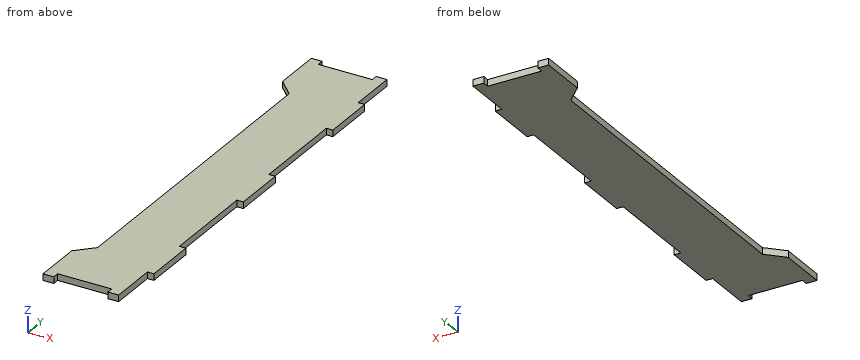
Autodesk Inventor part; units mm, degrees
ref_plane "YZ Plane" through (0, 0, 0) normal (1, 0, 0) x (0, 1, 0)
ref_plane "XZ Plane" through (0, 0, 0) normal (0, 1, 0) x (-1, 0, 0)
ref_plane "XY Plane" through (0, 0, 0) normal (0, 0, 1) x (1, 0, 0)
sketch "Sketch1" plane through (0, 0, 0) normal (0, 0, 1) x (1, 0, 0)
  line L0 (-6, 375) -> (0, 375) construction
  line L1 (0, 375) -> (0, 420) construction
  line L2 (0, 420) -> (-6, 420) construction
  line L3 (-6, 375) -> (-6, 420) construction
  line L4 (-6, 235) -> (0, 235) construction
  line L5 (0, 235) -> (0, 325) construction
  line L6 (0, 325) -> (-6, 325) construction
  line L7 (-6, 235) -> (-6, 325) construction
  line L8 (0, 185) -> (-6, 185) construction
  line L9 (-6, 95) -> (-6, 185) construction
  line L10 (-6, 95) -> (0, 95) construction
  line L11 (0, 95) -> (0, 185) construction
  line L12 (0, 45) -> (-6, 45) construction
  line L13 (-6, 0) -> (-6, 45) construction
  line L14 (0, 0) -> (-6, 0) construction
  line L15 (0, 0) -> (0, 45) construction
  line L16 (-6, 375) -> (0, 375)
  line L17 (0, 375) -> (0, 325)
  line L18 (0, 325) -> (-6, 325)
  line L19 (-6, 235) -> (0, 235)
  line L20 (0, 235) -> (0, 185)
  line L21 (0, 185) -> (-6, 185)
  line L22 (-6, 95) -> (0, 95)
  line L23 (0, 95) -> (0, 45)
  line L24 (0, 45) -> (-6, 45)
  line L25 (-6, 0) -> (-6, 45)
  line L26 (-6, 95) -> (-6, 185)
  line L27 (-6, 235) -> (-6, 325)
  line L28 (-6, 375) -> (-6, 420)
  line L29 (-76, 375) -> (-61, 375)
  line L30 (-61, 375) -> (-61, 45)
  line L31 (-61, 45) -> (-76, 45)
  line L32 (-76, 420) -> (-76, 375)
  line L33 (-76, 45) -> (-76, 0)
  line L34 (-66, 420) -> (-66, 414)
  line L35 (-66, 414) -> (-16, 414)
  line L36 (-16, 414) -> (-16, 420)
  line L37 (0, 210) -> (-61, 210) construction
  line L38 (-66, 0) -> (-66, 6)
  line L39 (-66, 6) -> (-16, 6)
  line L40 (-16, 6) -> (-16, 0)
  line L41 (-76, 0) -> (-66, 0)
  line L42 (-16, 0) -> (-6, 0)
  line L43 (-6, 420) -> (-16, 420)
  line L44 (-66, 420) -> (-76, 420)
  dimension "d0" = 70
  dimension "d1" = 15
  dimension "d2" = 50
  dimension "d3" = 6
  dimension "d4" = 10
extrude "Extrusion1" add sketch "Sketch1" against normal blind 6
chamfer "Chamfer1" distance 15 angle 45 2 edges at (-61, 375, -3) (-61, 45, -3)
properties part number "Frontal"
Source: CAD feature listing. Evaluate the final solid. Frame: model axes, mm. Give positions to 0.01 mm unless a question says otherwise; leave off trailing zeros. Order: outer loops, then holes, each group sorted by start corner. A loop starts at its lowest first (then second) coordinate and runs counter-clockwise, first axis right, second up. Notation, with made-up numbers: (5.5, 9) -> (10.5, 9) arc R25 cw to (10.5, 21) -> close; hole circle Ø4 at (-36, 64). An arc over 180 degrees is marked (long way). Write item = value, one per line.
Q1. Pin query (flat end, axial travel): pin 1 (3 mm diameter, centred on y = 417.5, z = -2.5, fed in from +X); pin 2 (1.8 mm diameter, centred on x = -3.5, z = -2, fed in from +Y). Return the tip coordinate at first contact, or that it passes through.
Data:
pin_1 = -6
pin_2 = 375
Q2. Cut plane C-C, the plane x = -34. Output: boundary loops of the cut face in (y, z).
Data:
outline = (6, -6) -> (414, -6) -> (414, 0) -> (6, 0) -> close
Q3. Material intervals for line 1 (X direction, y = 287, z = -3.5); line 2 (X direction, y = 189.5, z = -1.2); line 3 (Y direction, x = -43, z = -4.05), sorted ascending. Write a range as from..to.
Data:
line_1 = -61..-6
line_2 = -61..0
line_3 = 6..414
Q4. Cut plane B-B, the plane y = 196.5. Output: boundary loops of the cut face in (x, z).
Data:
outline = (-61, -6) -> (0, -6) -> (0, 0) -> (-61, 0) -> close
